Design review of the part built by this model. Coordinates are the model's own, in mm. Give positions to 0.01 mm unless a question says otherwise; leave off trailing zeros. Loops run counter-clockwise (first coordinate to the right, second up) from the corner with the lowest first, then second, coordinate; pieces in that order, holes last. Notation, with made-up numbers: (31, -19.75) - (55, -19.75) arc R23 ccw to (55, 6.25) - close; hole circle Ø2 at (-14, 67). An arc over 180 degrees is marked (long way). One line per item, written item: value. Start each with the question number.
```python
from build123d import *

# Parameters (mm, degrees)
F0_W          = 101.6
F0_H          = 101.6
F1_DEPTH      = 609.6
F2_R          = 12.7
F4_DEPTH      = 609.601
F4_DEPTH_BACK = 609.601
F6_D          = 13.49248


with BuildPart() as f1:
    # F0 (on Top) → F1 (new body, symmetric)
    with BuildSketch(Plane.XY):
        Rectangle(F0_W, F0_H)
    extrude(amount=F1_DEPTH, both=True)

    # F2
    f2_edges = [f1.edges().sort_by_distance(p)[0] for p in [
        (-50.8, 50.8, 0),
        (50.8, 50.8, 0),
        (50.8, -50.8, 0),
        (-50.8, -50.8, 0),
    ]]
    fillet(f2_edges, radius=F2_R)

    # F3 (on Top) → F4 (cut, two sides)
    with BuildSketch(Plane.XY) as f4_sk:
        with BuildLine():
            Line((38.1, 44.45), (-38.1, 44.45))
            ThreePointArc((-38.1, 44.45), (-42.5901280605, 42.5901280605), (-44.45, 38.1))
            Line((-44.45, 38.1), (-44.45, -38.1))
            ThreePointArc((-44.45, -38.1), (-42.5901280605, -42.5901280605), (-38.1, -44.45))
            Line((-38.1, -44.45), (38.1, -44.45))
            ThreePointArc((38.1, -44.45), (42.5901280605, -42.5901280605), (44.45, -38.1))
            Line((44.45, -38.1), (44.45, 38.1))
            ThreePointArc((44.45, 38.1), (42.5901280605, 42.5901280605), (38.1, 44.45))
        make_face()
    extrude(amount=-F4_DEPTH, mode=Mode.SUBTRACT)
    extrude(f4_sk.sketch, amount=F4_DEPTH_BACK, mode=Mode.SUBTRACT)

    # F6 (through all)
    with Locations(Plane.XZ.offset(50.8)):
        with Locations((0, 508), (0, 406.4)):
            Hole(F6_D / 2)


solid = f1.part
```
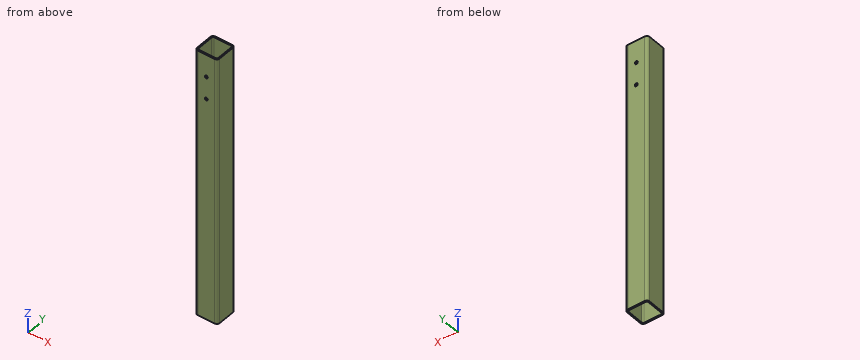
(1) To check wall thickness, follow L1, parallel to Z at x = 0, y = -46; L2, parallel to Y at x = -36, z = -499.5. State the ranges of each line that lie inside material, in increasing order. Write a range as from..to.
(2) Take a section at B-B on z = -163.5. State the section outline as (x, y) points, and give its area (3 significant figures).
(3) Take a section at A-A on y = -22.5. State the section outline as (x, z) points, and give its area (3 significant figures).
Here are the results:
1. L1: -609.6..399.65, 413.15..501.25, 514.75..609.6
1. L2: -50.8..-44.45, 44.45..50.8
2. outline: (-50.8, -38.1) arc R12.7 ccw to (-38.1, -50.8) - (38.1, -50.8) arc R12.7 ccw to (50.8, -38.1) - (50.8, 38.1) arc R12.7 ccw to (38.1, 50.8) - (-38.1, 50.8) arc R12.7 ccw to (-50.8, 38.1) - close; hole (-44.45, -38.1) arc R6.35 ccw to (-38.1, -44.45) - (38.1, -44.45) arc R6.35 ccw to (44.45, -38.1) - (44.45, 38.1) arc R6.35 ccw to (38.1, 44.45) - (-38.1, 44.45) arc R6.35 ccw to (-44.45, 38.1) - close
2. area: 2,320 mm²
3. outline: (-50.8, -609.6) - (-44.45, -609.6) - (-44.45, 609.6) - (-50.8, 609.6) - close; (44.45, -609.6) - (50.8, -609.6) - (50.8, 609.6) - (44.45, 609.6) - close
3. area: 15,500 mm²
